Design review of the part built by this model. Coordinates are the model's own, in mm. Give positions to 0.01 mm unless a question says otherwise; leave off trailing zeros. Order: outer loops, then holes, each group sorted by start corner. A loop starts at its lowest first (then second) coordinate and runs counter-clockwise, first axis right, second up. Notation, with made-up numbers: (43.5, 68.5) -> (72.5, 68.5) arc R22 cw to (72.5, 82.5) -> close; hole circle Ø10 at (43.5, 60). An arc over 180 degrees is marked (long way). Return JSON: item names as keys, results as strings.
```python
from build123d import *

# Parameters (mm, degrees)
F1_DEPTH = 10.16
F2_SIZE  = 5.07999


# Not quite as in the source:
# - a fillet or chamfer is up to 0.001 mm smaller than in the source, because OpenCascade refuses the exact size


with BuildPart() as f1:
    # F0 (on Right) → F1 (new body)
    with BuildSketch(Plane.YZ):
        Polygon((-45.6850975752, 0), (22.2317874432, -7.939924486), (22.2317874432, 0), align=None)
    extrude(amount=F1_DEPTH)

    # F2 (size 5.08 in the source; OpenCascade refuses exactly that, so slightly less here)
    f2_edges = [f1.edges().sort_by_distance(p)[0] for p in [
        (10.16, -11.726655, -3.969962),
        (0, -11.726655, -3.969962),
    ]]
    chamfer(f2_edges, length=F2_SIZE)


solid = f1.part
```
Item 1: Mouldability with a two-part tool opening along Y and no side actions: class faces 1 (the face through (5, 22.232, -3)), 2 (the face through (0, 15, -1)), 3 (the face through (3.07, -4.42, -2.8)) as released by +Y, released by -Y, zero draft, split by the parting line, or undercut.
Result set:
{"face 1": "released by +Y", "face 2": "zero draft", "face 3": "released by -Y"}
Item 2: For pin 1 (1.5 mm diameter, centred on x = 3.5, y = -3.5, fed in from -Z); pin 2 (2 mm diameter, centred on y = -11, z = -1.5, fed in from -X), all flat-tipped, find the tip position at first contact; note any pin that passes through.
Result set:
{"pin 1": "stops at z = -4.1", "pin 2": "stops at x = 1.54"}
Item 3: Add section C-C (x = 1.5). Give the boundary of the cut face in (y, z), plus the area to 3 significant figures.
Result set:
{"outline": "(-14.85, 0) -> (22.23, -4.34) -> (22.23, 0) -> close", "area": "80.4 mm^2"}
Item 4: Wall thickness on L1, parallel to Z at x = 6.5, y = 5.5; L2, parallel to Z at x = 7.5, y = -7.5; L3, parallel to X at y = -10.5, z = -1: over which ranges is each line inside the solid? List them lowest first. Write a range as [from, to].
Result set:
{"L1": "z = [-4.55, 0]", "L2": "z = [-2.03, 0]", "L3": "x = [1.99, 8.17]"}
Item 5: Add section D-D (x = 7.75). Give the boundary of the cut face in (y, z).
Result set:
{"outline": "(-22.69, 0) -> (22.23, -5.25) -> (22.23, 0) -> close"}
